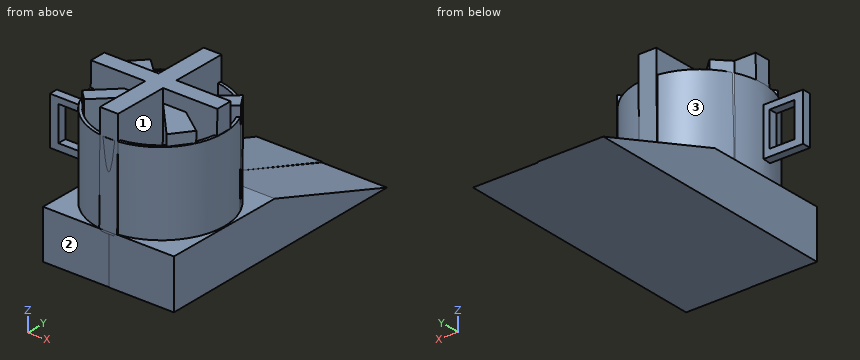
```python
from build123d import *
from build123d import SkipClean  # not in build123d's __all__

# Parameters (mm, degrees)
F0_W         = 53.0167296529
F0_H         = 70.1501816511
F2_W         = 33.9436382055
F2_H         = 39.762545377
F2_W_2       = 20.6894539297
F2_H_2       = 28.7712737918
F3_DEPTH     = 7.112
F4_T         = 2.54
F4_T3_DEPTH  = 44.842545377
F4_T5_DEPTH  = 12.192
F4_T8_ANGLE  = 7.7092595128
F4_T10_ANGLE = 7.7092595128
F6_DEPTH     = 54.102
F8_DEPTH     = 54.864
F9_W         = 14.9403763935
F9_H         = 46.2447360097
F9_W_2       = 45.0574515454
F9_H_2       = 13.7577369931
F10_DEPTH    = 88.646
F12_DEPTH    = 77.47


# Not quite as in the source:
# - a shell that OpenCascade refuses in one call is made with other operations: the cavity is built on its own and cut out


with BuildPart() as f1:
    # F0 (on Front) → F1 (revolve)
    with BuildSketch(Plane.XZ):
        with Locations((-26.5083648264, 0.9679794312)):
            Rectangle(F0_W, F0_H)
    revolve(axis=Axis((0, 0, 0.9679794312), (0, 0, 1)))

    # F2 (on Front) → F3 (join)
    with BuildSketch(Plane.XZ):
        with Locations((-69.0187290311, 0.6447080523)):
            Rectangle(F2_W, F2_H)
        with Locations((-68.5338173062, 0.9679803625)):
            Rectangle(F2_W_2, F2_H_2, mode=Mode.SUBTRACT)
    extrude(amount=F3_DEPTH)

    # F4: shell of thickness 2.54, made by hand


with BuildPart() as f4_core1:
    # F4_t2: copy of F1
    add(f1.part, clean=False)

    # the walls: a layer under each face that stays
    f4_faces = [f4_core1.faces().sort_by_distance(p)[0] for p in [
        (0, 0, -34.1071113944),
        (53.0167296529, 0, 0.9679794312),
        (-69.2640439234, -3.556, 20.5259807408),
        (-80.4150467304, -7.112, -12.6094737401),
        (-69.2640439234, -3.556, -19.2365646362),
        (-80.4949117204, 0, -12.6094737401),
        (-85.9905481339, -3.556, 0.6447080523),
        (-68.5338173062, -3.556, 15.3536172584),
        (-78.878544271, -3.556, 0.9679803625),
        (-58.1890903413, -3.556, 0.9679803625),
        (-68.5338173062, -3.556, -13.4176565334),
    ]]
    thicken(f4_faces, amount=-F4_T, mode=Mode.SUBTRACT)

    # F4_s4 → F4_t3 (cut)
    with BuildSketch(Plane.XY.offset(-21.7765646362)):
        Polygon((-52.5627101359, -7.1408073169), (-50.0204974181, -6.771268308), (-50.3182120863, -4.572), (-52.5375397129, -4.572), align=None)
        Polygon((-53.0421296529, 0.0254), (-50.4767296529, 0), (-50.4767296529, -2.54), (-53.0167296529, -2.54), align=None)
    extrude(amount=F4_T3_DEPTH, mode=Mode.SUBTRACT)

    # F4_s6 → F4_t5 (cut)
    with BuildSketch(Plane.XZ.offset(-2.54)):
        Polygon((-78.853144271, 15.3282172584), (-78.878544271, 17.8936172584), (-81.418544271, 17.8936172584), (-81.418544271, 15.3536172584), align=None)
        Polygon((-58.2144903413, 15.3282172584), (-58.1890903413, 17.8936172584), (-55.6490903413, 17.8936172584), (-55.6490903413, 15.3536172584), align=None)
        Polygon((-78.853144271, -13.3922565334), (-81.418544271, -13.4176565334), (-81.418544271, -15.9576565334), (-78.878544271, -15.9576565334), align=None)
        Polygon((-58.2144903413, -13.3922565334), (-55.6490903413, -13.4176565334), (-55.6490903413, -15.9576565334), (-58.1890903413, -15.9576565334), align=None)
    extrude(amount=F4_T5_DEPTH, mode=Mode.SUBTRACT)

    # F4_s7 → F4_t8 (revolve, cut)
    with BuildSketch(Plane(origin=(0, 0, 0), x_dir=(0, 0, 1), z_dir=(0.1341463354, -0.9909615334, 0))):
        Polygon((20.5513807408, 53.0421296529), (20.5259807408, 50.4767296529), (17.9859807408, 50.4767296529), (17.9859807408, 53.0167296529), align=None)
    revolve(axis=Axis((0, 0, 20.5259807408), (0, 0, -1)), revolution_arc=F4_T8_ANGLE, mode=Mode.SUBTRACT)

    # F4_s9 → F4_t10 (revolve, cut)
    with BuildSketch(Plane(origin=(0, 0, 0), x_dir=(0, 0, 1), z_dir=(0.1341463354, -0.9909615334, 0))):
        Polygon((-19.2619646362, 53.0421296529), (-19.2365646362, 50.4767296529), (-16.6965646362, 50.4767296529), (-16.6965646362, 53.0167296529), align=None)
    revolve(axis=Axis((0, 0, -19.2365646362), (0, 0, -1)), revolution_arc=F4_T10_ANGLE, mode=Mode.SUBTRACT)


with BuildPart() as f1_1:
    add(f1.part, clean=False)

    # what is left inside the walls is the cavity
    f4_cavity = [f4_core1.part.solids().sort_by_distance(p)[0] for p in [
        (50.3372, 3.391603, 13.506343),
    ]]
    add(f4_cavity, mode=Mode.SUBTRACT)

    # F5 (on Right) → F6 (join)
    with BuildSketch(Plane.YZ):
        Polygon((50.610627979, -33.1372953951), (-52.8366453946, -32.1674756706), (-52.8366453946, -73.2231140137), (165.6957119703, -73.2231140137), align=None)
    extrude(amount=F6_DEPTH)

    # F7 (on Right) → F8 (join)
    with BuildSketch(Plane.YZ):
        Polygon((52.1392673254, -33.7838381529), (-52.6010990143, -32.8140184283), (-52.6010990143, -73.2231140137), (166.5778160095, -73.2231140137), align=None)
    extrude(amount=-F8_DEPTH)

    # F9 (on face) → F10 (join)
    with BuildSketch(Plane(origin=(0, -0.3061875117, -32.6599494936), x_dir=(1, 0, 0), z_dir=(0, 0.0093746029, 0.9999560574))):
        with Locations((0, -30.0012365014)):
            Rectangle(F9_W, F9_H)
        with Locations((-29.9989139694, 0)):
            Rectangle(F9_W_2, F9_H_2)
        Rectangle(F9_W, F9_H_2)
        with Locations((29.9989139694, 0)):
            Rectangle(F9_W_2, F9_H_2)
        with Locations((0, 30.0012365014)):
            Rectangle(F9_W, F9_H)
    with SkipClean():  # cleaning this boolean's faces spoils the solid; the shape is the same uncleaned
        extrude(amount=F10_DEPTH)

    # F11 (on face) → F12 (join)
    with BuildSketch(Plane(origin=(0, -0.3061875117, -32.6599494936), x_dir=(1, 0, 0), z_dir=(0, 0.0093746029, 0.9999560574))):
        Polygon((-35.2792814374, -35.0489541888), (-6.9552087225, -6.723633036), (7.4701881967, -6.8788684965), (-9.015141055, 8.7265400216), (-36.82423383, 34.9918417633), (-47.9992774731, 23.1599645401), (-27.8100166411, 4.0914881974), (-22.4047969755, -4.6636964383), (-44.0343843394, -26.2942371678), align=None)
        Polygon((9.0424474554, 7.2099834745), (7.4701881967, -6.8788684965), (36.0927975577, -38.5295574829), (47.8385306477, -22.5475626063), (26.5187043697, -6.8788684965), (26.5187043697, 4.0914881974), (47.8385306477, 23.1599645401), (40.2370781386, 34.8294671803), align=None)
        Polygon((-9.015141055, 8.7265400216), (7.4701881967, -6.8788684965), (9.0424474554, 7.2099834745), align=None)
    with SkipClean():  # cleaning this boolean's faces spoils the solid; the shape is the same uncleaned
        extrude(amount=F12_DEPTH)


solid = f1_1.part
```
Here's how the part is built. I have some questions about the finished solid (model axes, mm). Face numbers are marked on the shaded views. Round coordinates to 2 decimals unless told otherwise and drop trailing zeros. Order: outer loops, then holes, each group sorted by start corner. A loop starts at its lowest first (then second) coordinate and runs counter-clockwise, first axis right, second up. Notation, with made-up numbers: M -11,10 L 7,10 A28 ccw 7,43 Z; hole C 3,85.25 d7. An arc over 180 degrees is marked long. Answer in a Markdown table with one row per item.
Item 1: Imagine slicing it at D-D, the plane x = -12. Write out the boundary of the cut face in (y, z).
A:
| item | result |
|---|---|
| outline | M -52.6,-73.22 L 166.58,-73.22 L 52.14,-33.78 L 51.64,-33.78 L 51.64,36.04 L 49.03,36.04 L 49.03,-31.57 L 11.25,-31.57 L 11.97,44.7 L 7.3,44.74 L 7.4,55.92 L -6.35,56.05 L -6.46,44.87 L -11.35,44.92 L -12.07,-31.57 L -49.03,-31.57 L -49.03,36.04 L -51.64,36.04 L -51.64,-32.82 L -52.6,-32.81 Z |
Item 2: Imagine slicing it at A-A, the plane x = -76.5. Write out the boundary of the cut face in (y, z).
A:
| item | result |
|---|---|
| outline | M -7.11,-19.24 L 0,-19.24 L 0,-13.42 L -7.11,-13.42 Z; M -7.11,15.35 L 0,15.35 L 0,20.53 L -7.11,20.53 Z; hole M -4.57,-16.7 L -2.54,-16.7 L -2.54,-15.96 L -4.57,-15.96 Z; hole M -4.57,17.89 L -2.54,17.89 L -2.54,17.99 L -4.57,17.99 Z |
Item 3: Imagine slicing it at B-B, the plane z = 7. State how many separate pieces and enclosed holes the cut face has, and give its area (3 significant figures).
A:
| item | result |
|---|---|
| separate pieces | 2 |
| enclosed holes | 10 |
| area | 5,480 mm2 |
Item 4: Thinking about a two-plate mould opening in X: for the marked faces 1, 2 and 3, which applies, +X half, -X half, draft (parallel to the pull), parting line (faces both ways), or undercut?
A:
| item | result |
|---|---|
| face 1 | undercut |
| face 2 | draft |
| face 3 | parting line |
Item 5: I'm going to push flat-ended pins straight in: pin 1 (5 mm diameter, centred on x = -28.5, y = 110.5, fed in from +Z); pin 2 (8 mm diameter, centred on x = -71.5, y = -4.5, fed in from +Z); pin 3 (23.5 mm diameter, centred on y = -20, z = 13, fed in from -X). Where does each tip first touch, or does it pass through?
A:
| item | result |
|---|---|
| pin 1 | stops at z = -53.04 |
| pin 2 | stops at z = 20.53 |
| pin 3 | stops at x = -52.37 |
Item 6: If I drill on L1, parallel to X at y = -13, z = -7; L2, parallel to Y at x = -39, z = -15.5; L3, parallel to Y at x = -43, z = 9, over which ranges is the centre line in solid material (lowest first)? Write a range as from..to.
A:
| item | result |
|---|---|
| L1 | x = -51.4..-48.77, -30.67..-13.17, -7.47..7.47, 12.95..34.76, 48.77..51.4 |
| L2 | y = -35.91..-32.05, -31.48..-21.41, -7.02..6.73, 14.52..35.91 |
| L3 | y = -31.01..-25.18, -6.79..6.96, 18.52..31.01 |
Item 7: Imagine slicing it at C-C, the plane y = 28.5. Write out the boundary of the cut face in (x, z), and give its area (3 significant figures).
A:
| item | result |
|---|---|
| outline | M -54.86,-73.22 L 54.1,-73.22 L 54.1,-32.93 L 44.7,-32.93 L 44.7,36.04 L 44.58,36.04 L 44.63,44.54 L 32.62,44.54 L 33.42,-31.57 L 7.47,-31.57 L 7.47,55.72 L -7.47,55.72 L -7.47,-31.57 L -30.26,-31.57 L -29.51,44.54 L -43.35,44.54 L -43.28,36.04 L -44.7,36.04 L -44.7,-33.56 L -54.86,-33.56 Z |
| area | 7,810 mm2 |
